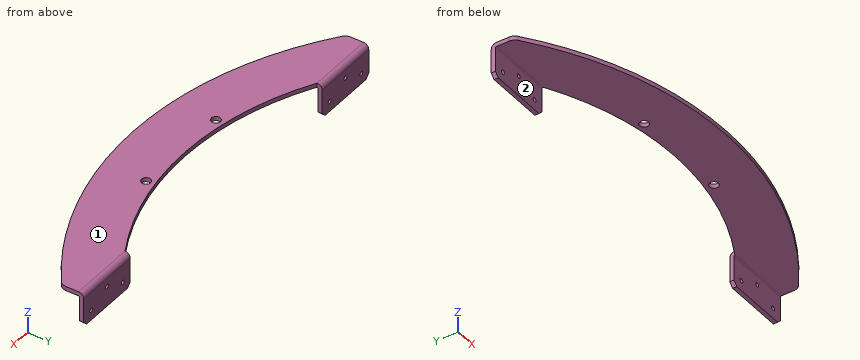
```python
from build123d import *

# Parameters (mm, degrees)
BASE_FLANGE1_DEPTH        = 3.175
EDGE_FLANGE1_DEPTH        = 50.8
EDGE_FLANGE1_BEND_DEPTH   = 50.8
SKETCH25_R                = 3.3782
CUT_EXTRUDE1_DEPTH        = 320.039055649
BREAK_CORNER1_START       = 15.715448212
BREAK_CORNER1_OUTLINE_W   = 184.095250482
BREAK_CORNER1_OUTLINE_H   = 6
BREAK_CORNER1_DEPTH       = 152.664354058
BREAK_CORNER1_START_2     = -17.960512242
BREAK_CORNER1_2_OUTLINE_W = 37.636472696
BREAK_CORNER1_2_OUTLINE_H = 6
BREAK_CORNER1_2_DEPTH     = 2.24506403
BREAK_CORNER1_START_3     = 199.810698694
BREAK_CORNER1_3_OUTLINE_W = 2.268276822
BREAK_CORNER1_3_OUTLINE_H = 6
BREAK_CORNER1_3_DEPTH     = 4.49012806
SKETCH26_R                = 1.5875
CUT_EXTRUDE2_DEPTH        = 320.868403774
SKETCH27_R                = 1.5875
CUT_EXTRUDE3_DEPTH        = 320.868403774


# Read off the part's stored shape, not the designer's step: Break-Corner1
# Sheet-metal steps are written as plain solids
with BuildPart() as part:
    # Sketch2 → Base-Flange1 (new body)
    with BuildSketch(Plane.XY):
        with BuildLine():
            Line((0, 0), (50.8, 0))
            ThreePointArc((50.8, 0), (155.575, -27.127625498), (260.35, 0))
            Line((260.35, 0), (311.15, 0))
            Line((311.15, 0), (311.15, -9.556040603))
            ThreePointArc((311.15, -9.556040603), (310.481801777, -12.39146448), (308.617833524, -14.630156012))
            ThreePointArc((308.617833524, -14.630156012), (155.575, -65.775653014), (2.532166476, -14.630156012))
            ThreePointArc((2.532166476, -14.630156012), (0.668198223, -12.39146448), (0, -9.556040603))
            Line((0, -9.556040603), (0, 0))
        make_face()
    extrude(amount=-BASE_FLANGE1_DEPTH)

    # Edge-Flange1 section (across the edge) → Edge-Flange1 (add)
    with BuildSketch(Plane(origin=(0, 0.7366, -3.175), x_dir=(0, -1, 0), z_dir=(1, 0, 0))):
        with BuildLine():
            Line((-3.175, 0.7366), (-3.175, 22.225))
            Line((-3.175, 22.225), (0, 22.225))
            Line((0, 22.225), (0, 0.7366))
            ThreePointArc((0, 0.7366), (0.215745145, 0.215745145), (0.7366, 0))
            Line((0.7366, 0), (0.7366, -3.175))
            ThreePointArc((0.7366, -3.175), (-2.029318885, -2.029318885), (-3.175, 0.7366))
        make_face()
    extrude(amount=EDGE_FLANGE1_DEPTH)

    # Edge-Flange1 section 2 (across the edge) → Edge-Flange1 bend (add)
    with BuildSketch(Plane(origin=(260.35, 0.7366, -3.175), x_dir=(0, -1, 0), z_dir=(1, 0, 0))):
        with BuildLine():
            Line((-3.175, 0.7366), (-3.175, 22.225))
            Line((-3.175, 22.225), (0, 22.225))
            Line((0, 22.225), (0, 0.7366))
            ThreePointArc((0, 0.7366), (0.215745145, 0.215745145), (0.7366, 0))
            Line((0.7366, 0), (0.7366, -3.175))
            ThreePointArc((0.7366, -3.175), (-2.029318885, -2.029318885), (-3.175, 0.7366))
        make_face()
    extrude(amount=EDGE_FLANGE1_BEND_DEPTH)

    # Sketch25 → Cut-Extrude1 (cut, through all)
    with BuildSketch(Plane.XY):
        with Locations((117.475, -30.187559048)):
            Circle(SKETCH25_R)
        with Locations((193.675, -30.187559048)):
            Circle(SKETCH25_R)
    extrude(amount=-CUT_EXTRUDE1_DEPTH, mode=Mode.SUBTRACT)

    # Break-Corner1 outline → Break-Corner1 (cut)
    with BuildSketch(Plane(origin=(0, 0, 0), x_dir=(0.707106781186548, 0, -0.707106781186547), z_dir=(0.707106781186547, 0, 0.707106781186548)).offset(BREAK_CORNER1_START)):
        with Locations((143.684097937, 2)):
            Rectangle(BREAK_CORNER1_OUTLINE_W, BREAK_CORNER1_OUTLINE_H)
    extrude(amount=BREAK_CORNER1_DEPTH, mode=Mode.SUBTRACT)

    # Break-Corner1 2 outline → Break-Corner1 2 (cut)
    with BuildSketch(Plane(origin=(0, 0, 0), x_dir=(0.707106781186548, 0, -0.707106781186547), z_dir=(0.707106781186547, 0, 0.707106781186548)).offset(BREAK_CORNER1_START_2)):
        with Locations((32.818236348, 2)):
            Rectangle(BREAK_CORNER1_2_OUTLINE_W, BREAK_CORNER1_2_OUTLINE_H)
    extrude(amount=BREAK_CORNER1_2_DEPTH, mode=Mode.SUBTRACT)

    # Break-Corner1 3 outline → Break-Corner1 3 (cut)
    with BuildSketch(Plane(origin=(0, 0, 0), x_dir=(0.707106781186548, 0, -0.707106781186547), z_dir=(0.707106781186547, 0, 0.707106781186548)).offset(BREAK_CORNER1_START_3)):
        with Locations((236.865861589, 2)):
            Rectangle(BREAK_CORNER1_3_OUTLINE_W, BREAK_CORNER1_3_OUTLINE_H)
    extrude(amount=BREAK_CORNER1_3_DEPTH, mode=Mode.SUBTRACT)

    # Sketch26 → Cut-Extrude2 (cut, through all)
    with BuildSketch(Plane(origin=(0, 3.9116, 0), x_dir=(1, 0, 0), z_dir=(0, 1, 0))):
        with Locations(Location((8.128, 17.78, 0), (0, 0, 270))):
            Circle(SKETCH26_R)
        with Locations(Location((25.4, 10.16, 0), (0, 0, 270))):
            Circle(SKETCH26_R)
        with Locations(Location((42.672, 17.78, 0), (0, 0, 270))):
            Circle(SKETCH26_R)
    extrude(amount=-CUT_EXTRUDE2_DEPTH, mode=Mode.SUBTRACT)

    # Sketch27 → Cut-Extrude3 (cut, through all)
    with BuildSketch(Plane(origin=(0, 3.9116, 0), x_dir=(1, 0, 0), z_dir=(0, 1, 0))):
        with Locations(Location((268.478, 17.78, 0), (0, 0, 270))):
            Circle(SKETCH27_R)
        with Locations(Location((303.022, 17.78, 0), (0, 0, 270))):
            Circle(SKETCH27_R)
        with Locations(Location((285.75, 10.16, 0), (0, 0, 270))):
            Circle(SKETCH27_R)
    extrude(amount=-CUT_EXTRUDE3_DEPTH, mode=Mode.SUBTRACT)


solid = part.part
```
Read the model definition and answer for the solid it produces. Units are mm, in the model's axes. Face numbers are marked on the shaded views. A direction names the side the tool comes from. Give positions to 0.01 mm unless a question says otherwise; leave off trailing zeros. Order: outer loops, then holes, each group sorted by start corner. A loop starts at its lowest first (then second) coordinate and runs counter-clockwise, first axis right, second up. Notation, with made-up numbers: (12, -15) -> (47, -15) arc R24 ccw to (47, -3) -> close; hole circle Ø11 at (36.5, 63.5). An arc over 180 degrees is marked (long way). One line per item, written item: value. Start each with the question number.
(1) Straight lines are drawn through the part: L1, parallel to X at y = 1.85, z = -17.78; L2, parallel to Z at x = 165.5, y = -47 (3 decimals); L3, parallel to Y at x = 32, z = -12. For each, find the intervals that lie inside material, in ascending order.
(2) The part is cut by section B-B (x = 143.5). Determine the outline of the cut face in (y, z) (3 decimals), and give its area (3 significant figures).
(3) Flat-ended cylindrical pins translate along their axes: P1, Ø6, axis at x = 193.68, y = -30.19, coming from the +Z side; P2, Ø8, axis at x = 117.48, y = -30.19, coming from the -Z side (3 decimals); P3, Ø3.5, axis at x = 303.022, z = -17.78, coming from the -Y side. Find the tip coordinate at first contact, or state that the pin passes through.
(4) The part is cut by section A-A (y = -59). Determine the outline of the cut face in (x, z) (3 decimals).
(5) A tool of negligible diameter and unlimited length cuts with its end or side. For the marked faces 1 and 2, from which of +Z, -Z, +X, -X, +Y, -Y can it reach the whole face along a straight path? Write none if from no direction.
Taken from the geometry:
1. L1: 0 to 6.54, 9.72 to 41.08, 44.26 to 50.8, 260.35 to 266.89, 270.07 to 301.43, 304.61 to 311.15
1. L2: -3.175 to 0
1. L3: 0.74 to 3.91
2. outline: (-65.489, -3.175) -> (-26.79, -3.175) -> (-26.79, 0) -> (-65.489, 0) -> close
2. area: 123 mm^2
3. P1: through
3. P2: z = -3.175
3. P3: y = 0.74
4. outline: (97.235, -3.175) -> (213.915, -3.175) -> (213.915, 0) -> (97.235, 0) -> close
5. face 1: +Z, +X, -X, +Y, -Y
5. face 2: -Z, +X, -X, -Y
